Work out the finished part from the listing and answer in its coordinate system (mm). A direction names the side the tool comes from. Give positions to 0.01 mm unless a question says otherwise; leave off trailing zeros. Loops run counter-clockwise (first coordinate to the right, second up) from the corner with the lowest first, then second, coordinate; pieces in that order, holes last. Notation, with made-up numbers: (10, 32) - (49, 32) arc R12 cw to (49, 43) - close; hole circle Ø5 at (76, 82.25). An arc over 180 degrees is marked (long way). Use one line per item in the form item = value. Start each with the question number.
Autodesk Inventor part; units mm, degrees
ref_plane "YZ Plane" through (0, 0, 0) normal (1, 0, 0) x (0, 1, 0)
ref_plane "XZ Plane" through (0, 0, 0) normal (0, 1, 0) x (-1, 0, 0)
ref_plane "XY Plane" through (0, 0, 0) normal (0, 0, 1) x (1, 0, 0)
sketch "Sketch1" plane through (0, 0, 0) normal (0, 0, 1) x (1, 0, 0)
  line L0 (0, 0) -> (12.7, 0)
  line L1 (12.7, 0) -> (12.7, 38.1)
  line L2 (12.7, 38.1) -> (0, 38.1)
  line L3 (0, 38.1) -> (0, 0)
  dimension "d0" = 38.1
  dimension "d1" = 12.7
extrude "Extrusion1" add sketch "Sketch1" along normal blind 152.4
shell "Shell1" thickness 1.27 removed faces 2 at (4.2333, 25.4, 0) at (4.2333, 25.4, 152.4)
sketch "Sketch2" plane through (12.7, 0, 0) normal (1, 0, 0) x (0, 0, -1)
  line L0 (0, 0) -> (0, 38.1)
  line L1 (0, 38.1) -> (-152.4, 38.1)
  line L2 (-152.4, 0) -> (-152.4, 38.1)
  line L3 (0, 0) -> (-152.4, 0)
  line L4 (-162.6393, 19.05) -> (14.976, 19.05) construction
  point P0 (-133.35, 19.05)
  point P1 (-19.05, 19.05)
  dimension "d5" = 19.05
  dimension "d6" = 19.05
  dimension "d9" = 19.05
hole "Hole1" at (12.7, 19.05, 133.35) at (12.7, 19.05, 19.05) direction (-1, 0, 0) diameter 7.112 end through all
sketch "Sketch3" plane through (0, 38.1, 0) normal (0, 1, 0) x (1, 0, 0)
  line L0 (12.7, 0) -> (0, 0)
  line L1 (0, 0) -> (0, -152.4)
  line L2 (12.7, -152.4) -> (0, -152.4)
  line L3 (12.7, 0) -> (12.7, -152.4)
  line L4 (6.35, 17.6784) -> (6.35, -171.0582) construction
  point P0 (0, 0)
  point P1 (6.35, -25.4)
  point P2 (6.35, -127)
  point P3 (6.35, -76.2)
  dimension "d17" = 6.35
  dimension "d18" = 25.4
  dimension "d19" = 25.4
  dimension "d20" = 76.2
hole "Hole2" at (6.35, 38.1, 25.4) at (6.35, 38.1, 127) at (6.35, 38.1, 76.2) direction (0, -1, 0) diameter 7.112 end through all
properties part number "090000-1"
1) A cutting plane is placed at B-B (z = 25.4). Give the vertices of the cut face in (x, y).
2) A cutting plane is placed at C-C (x = 6.35). State how many separate pieces and enclosed holes the cut face has, plus the area to 3 significant figures.
3) A tool of negligible diameter and unlimited length cuts with its end or side. For faces 1 (the flat face through (10, 36.83, 75)), 2 (the flat face through (10, 0, 75)), from which of +Z, -Z, +X, -X, +Y, -Y can it reach the whole face along a straight path? Write none if from no direction.
4) Find the intervals of material crossed by probe 1 along Z at (x, y) = (6.35, 37.5); probe 2 along Z at (x, y) = (0.75, 19.05); probe 3 along X at (y, z) = (20, 114), in increasing order.
5) A cutting plane is placed at A-A (y = 19.05). Give the vertices of the cut face in (x, z), plus the area to 3 significant figures.
6) Determine the mould class of faces 3 (the cylindrical face through (6.194, 37.456, 123.447)), 4 (the flat face through (2, 38.1, 75)), 5 (the flat face through (2, 1.27, 75)) for opening direction Y: released by +Y, released by -Y, zero draft, split by the parting line, or undercut.
7) A cutting plane is placed at D-D (z = 102.5). Give the vertices of the cut face in (x, y), plus the area to 3 significant figures.
Answer sheet:
q1.outline = (0, 0) - (2.79, 0) - (2.79, 1.27) - (1.27, 1.27) - (1.27, 36.83) - (2.79, 36.83) - (2.79, 38.1) - (0, 38.1) - close; (9.91, 0) - (12.7, 0) - (12.7, 38.1) - (9.91, 38.1) - (9.91, 36.83) - (11.43, 36.83) - (11.43, 1.27) - (9.91, 1.27) - close
q2.separate_pieces = 8
q2.enclosed_holes = 0
q2.area = 333 mm²
q3.face_1 = +Z, -Z
q3.face_2 = +Z, -Z, +X, -X, -Y
q4.probe_1 = 0 to 21.84, 28.96 to 72.64, 79.76 to 123.44, 130.56 to 152.4
q4.probe_2 = 0 to 15.49, 22.61 to 129.79, 136.91 to 152.4
q4.probe_3 = 0 to 1.27, 11.43 to 12.7
q5.outline = (0, 0) - (1.27, 0) - (1.27, 15.49) - (0, 15.49) - close; (0, 22.61) - (1.27, 22.61) - (1.27, 129.79) - (0, 129.79) - close; (0, 136.91) - (1.27, 136.91) - (1.27, 152.4) - (0, 152.4) - close; (11.43, 0) - (12.7, 0) - (12.7, 15.49) - (11.43, 15.49) - close; (11.43, 22.61) - (12.7, 22.61) - (12.7, 129.79) - (11.43, 129.79) - close; (11.43, 136.91) - (12.7, 136.91) - (12.7, 152.4) - (11.43, 152.4) - close
q5.area = 351 mm²
q6.face_3 = zero draft
q6.face_4 = released by +Y
q6.face_5 = undercut
q7.outline = (0, 0) - (12.7, 0) - (12.7, 38.1) - (0, 38.1) - close; hole (1.27, 1.27) - (11.43, 1.27) - (11.43, 36.83) - (1.27, 36.83) - close
q7.area = 123 mm²
